```python
from build123d import *

# Parameters (mm, degrees)
SKETCH_1_R                  = 0.95
EXTRUDE_1_DEPTH             = 1.8
FILLET_1_R                  = 2
HOLE_WIZARD_M2_1_AT_2_COUNT = 2
HOLE_WIZARD_M2_1_AT_2_PITCH = 24
HOLE_WIZARD_M2_1_AT_3_COUNT = 2
HOLE_WIZARD_M2_1_AT_3_PITCH = 39.40177661
HOLE_WIZARD_M2_1_AT_4_COUNT = 2
HOLE_WIZARD_M2_1_AT_4_PITCH = 45
HOLE_WIZARD_M2_1_AT_5_COUNT = 2
HOLE_WIZARD_M2_1_AT_5_PITCH = 38.065732621
HOLE_WIZARD_M2_1_AT_6_COUNT = 2
HOLE_WIZARD_M2_1_AT_6_PITCH = 21.737065119
SKETCH_4_R                  = 17.25
SKETCH_4_R_2                = 15
EXTRUDE_2_DEPTH             = 4.2
SKETCH_4_2_R                = 15
CUT_EXTRUDE_2_DEPTH         = 3.5
SKETCH_7_R                  = 0.85
EXTRUDE_3_DEPTH             = 6
SKETCH_7_2_R                = 0.85
CUT_EXTRUDE_4_DEPTH         = 7
SKETCH_8_R                  = 4
CUT_EXTRUDE_5_DEPTH         = 10


with BuildPart() as part:
    # Sketch 1 → Extrude 1 (new body)
    with BuildSketch(Plane(origin=(0, 0, 0), x_dir=(1, 0, 0), z_dir=(0, 1, 0))):
        Polygon((33, 0), (16.5, 28.578838325), (-16.5, 28.578838325), (-33, 0), (-16.5, -28.578838325), (16.5, -28.578838325), align=None)
        with Locations(Location((-12, 19.032866311, 0), (0, 0, 270))):  # turned: the seam where the file's is
            Circle(SKETCH_1_R, mode=Mode.SUBTRACT)
        with Locations(Location((-12, -19.032866311, 0), (0, 0, 90))):  # turned: the seam where the file's is
            Circle(SKETCH_1_R, mode=Mode.SUBTRACT)
        with Locations(Location((-22.5, 0, 0), (0, 0, 270))):  # turned: the seam where the file's is
            Circle(SKETCH_1_R, mode=Mode.SUBTRACT)
        with Locations(Location((22.5, 0, 0), (0, 0, 90))):  # turned: the seam where the file's is
            Circle(SKETCH_1_R, mode=Mode.SUBTRACT)
        with Locations(Location((12, -19.032866311, 0), (0, 0, 270))):  # turned: the seam where the file's is
            Circle(SKETCH_1_R, mode=Mode.SUBTRACT)
        with Locations(Location((12, 19.032866311, 0), (0, 0, 90))):  # turned: the seam where the file's is
            Circle(SKETCH_1_R, mode=Mode.SUBTRACT)
    extrude(amount=EXTRUDE_1_DEPTH)

    # Fillet 1
    fillet_1_edges = [part.edges().sort_by_distance(p)[0] for p in [
        (16.5, 0.9, 28.578838325),
        (-16.5, 0.9, 28.578838325),
        (-33, 0.9, 0),
        (-16.5, 0.9, -28.578838325),
        (16.5, 0.9, -28.578838325),
        (33, 0.9, 0),
    ]]
    fillet(fillet_1_edges, radius=FILLET_1_R)

    # Sketch 3 → Hole Wizard M2 _1 (revolve, cut)
    with BuildSketch(Plane(origin=(12, 0, -19.032866311), x_dir=(0, 0, -1), z_dir=(1, 0, 0))):
        Polygon((0, 0), (0, 1.8), (0.9, 1.8), (0.9, 1.2), (2.1, 0), align=None)
    hole_wizard_m2_1 = revolve(axis=Axis((12, -6.35, -19.032866311), (0, 1, 0)), mode=Mode.SUBTRACT)

    # Hole Wizard M2 _1 at 2: Hole Wizard M2 _1 ×2
    with Locations(*[(-i * HOLE_WIZARD_M2_1_AT_2_PITCH, 0, 0) for i in range(1, HOLE_WIZARD_M2_1_AT_2_COUNT)]):
        add(hole_wizard_m2_1, mode=Mode.SUBTRACT)

    # Hole Wizard M2 _1 at 3: Hole Wizard M2 _1 ×2
    with Locations(*[Vector(-0.875595036, 0, 0.483045892) * (i * HOLE_WIZARD_M2_1_AT_3_PITCH) for i in range(1, HOLE_WIZARD_M2_1_AT_3_COUNT)]):
        add(hole_wizard_m2_1, mode=Mode.SUBTRACT)

    # Hole Wizard M2 _1 at 4: Hole Wizard M2 _1 ×2
    with Locations(*[Vector(-0.533333333, 0, 0.845905169) * (i * HOLE_WIZARD_M2_1_AT_4_PITCH) for i in range(1, HOLE_WIZARD_M2_1_AT_4_COUNT)]):
        add(hole_wizard_m2_1, mode=Mode.SUBTRACT)

    # Hole Wizard M2 _1 at 5: Hole Wizard M2 _1 ×2
    with Locations(*[(0, 0, i * HOLE_WIZARD_M2_1_AT_5_PITCH) for i in range(1, HOLE_WIZARD_M2_1_AT_5_COUNT)]):
        add(hole_wizard_m2_1, mode=Mode.SUBTRACT)

    # Hole Wizard M2 _1 at 6: Hole Wizard M2 _1 ×2
    with Locations(*[Vector(0.483045892, 0, 0.875595036) * (i * HOLE_WIZARD_M2_1_AT_6_PITCH) for i in range(1, HOLE_WIZARD_M2_1_AT_6_COUNT)]):
        add(hole_wizard_m2_1, mode=Mode.SUBTRACT)

    # Sketch 4 → Extrude 2 (add)
    with BuildSketch(Plane.XZ):
        with Locations(Location((0, 0, 0), (0, 0, 90))):  # turned: the seam where the file's is
            Circle(SKETCH_4_R)
        with Locations(Location((0, 0, 0), (0, 0, 270))):  # turned: the seam where the file's is
            Circle(SKETCH_4_R_2, mode=Mode.SUBTRACT)
    extrude(amount=EXTRUDE_2_DEPTH)

    # Sketch 4_2 → Cut-Extrude 2 (cut)
    with BuildSketch(Plane.XZ):
        with Locations(Location((0, 0, 0), (0, 0, 90))):  # turned: the seam where the file's is
            Circle(SKETCH_4_2_R)
    extrude(amount=-CUT_EXTRUDE_2_DEPTH, mode=Mode.SUBTRACT)

    # Sketch 7 → Extrude 3 (add)
    with BuildSketch(Plane.XZ.offset(4.2)):
        with BuildLine():
            ThreePointArc((-13.77195188, 10.387292305), (-9.652159983, 8.099123882), (-12.620960341, 11.758990606))
            ThreePointArc((-12.620960341, 11.758990606), (-13.214266644, 11.088086267), (-13.77195188, 10.387292305))
        make_face()
        with Locations((-11.490666647, 9.641814145)):
            Circle(SKETCH_7_R, mode=Mode.SUBTRACT)
        with BuildLine():
            ThreePointArc((13.77195188, 10.387292305), (9.652159983, 8.099123882), (12.620960341, 11.758990606))
            ThreePointArc((12.620960341, 11.758990606), (13.214266644, 11.088086267), (13.77195188, 10.387292305))
        make_face()
        with Locations((11.490666647, 9.641814145)):
            Circle(SKETCH_7_R, mode=Mode.SUBTRACT)
        with BuildLine():
            ThreePointArc((13.77195188, -10.387292305), (9.652159983, -8.099123882), (12.620960341, -11.758990606))
            ThreePointArc((12.620960341, -11.758990606), (13.214266644, -11.088086267), (13.77195188, -10.387292305))
        make_face()
        with Locations((11.490666647, -9.641814145)):
            Circle(SKETCH_7_R, mode=Mode.SUBTRACT)
        with BuildLine():
            ThreePointArc((-13.77195188, -10.387292305), (-9.652159983, -8.099123882), (-12.620960341, -11.758990606))
            ThreePointArc((-12.620960341, -11.758990606), (-13.214266644, -11.088086267), (-13.77195188, -10.387292305))
        make_face()
        with Locations((-11.490666647, -9.641814145)):
            Circle(SKETCH_7_R, mode=Mode.SUBTRACT)
    extrude(amount=-EXTRUDE_3_DEPTH)

    # Sketch 7_2 → Cut-Extrude 4 (cut, through all)
    with BuildSketch(Plane.XZ.offset(4.2)):
        with Locations(Location((-11.490666647, 9.641814145, 0), (0, 0, 270))):  # turned: the seam where the file's is
            Circle(SKETCH_7_2_R)
        with Locations(Location((11.490666647, 9.641814145, 0), (0, 0, 90))):  # turned: the seam where the file's is
            Circle(SKETCH_7_2_R)
        with Locations(Location((11.490666647, -9.641814145, 0), (0, 0, 270))):  # turned: the seam where the file's is
            Circle(SKETCH_7_2_R)
        with Locations(Location((-11.490666647, -9.641814145, 0), (0, 0, 90))):  # turned: the seam where the file's is
            Circle(SKETCH_7_2_R)
    extrude(amount=-CUT_EXTRUDE_4_DEPTH, mode=Mode.SUBTRACT)

    # Sketch 8 → Cut-Extrude 5 (cut)
    with BuildSketch(Plane(origin=(0, 1.8, 0), x_dir=(1, 0, 0), z_dir=(0, 1, 0))):
        with Locations(Location((-23.2, 0, 0), (0, 0, 270))):  # turned: the seam where the file's is
            Circle(SKETCH_8_R)
    extrude(amount=-CUT_EXTRUDE_5_DEPTH, mode=Mode.SUBTRACT)


solid = part.part
```
Work out the finished part from the listing and answer in its coordinate system (mm). A direction names the side the tool comes from. Coordinates: 2 decimals unless noted, no trailing zeros. Loops run counter-clockwise (first coordinate to the right, second up) from the corner with the lowest first, then second, coordinate; pieces in that order, holes last.
1) Flat-ended cylindrical pins translate along their axes: pin 1 (2.5 mm diameter, centred on x = 12, z = -19.03, fed in from -Y); pin 2 (2 mm diameter, centred on x = 22.5, z = 0, fed in from -Y); pin 3 (1.4 mm diameter, centred on x = -11.49, z = -9.64, fed in from -Y); pin 4 (3 mm diameter, centred on x = 7.5, y = -2, fed in from +Z). Find the tip coordinate at first contact, or state that the pin passes through.
Results:
pin 1: stops at y = 0.85
pin 2: stops at y = 1.1
pin 3: passes through
pin 4: stops at z = 16.17
2) For faces 5 (the cylindrical face through (16.36, 0.91, -28.3)), 6 (the flat face through (14, 0, 12)), 7 (the cylindrical face through (0, -1, -15)), determine the directions among +Z, -Z, +X, -X, +Y, -Y from which every point of the face is accessible in a straight line to the end or side of a thin tool.
Results:
face 5: -Z, +X, +Y, -Y
face 6: -Y
face 7: +Y, -Y
3) Section A-A (z = 13) is taken. Give the vertices of the cut face in (x, y), plus the area to 3 significant figures.
Results:
outline: (-25.49, 0) - (-11.34, 0) - (-11.34, -4.2) - (-7.48, -4.2) - (-7.48, 1.8) - (-25.49, 1.8) - close; (7.48, -4.2) - (11.34, -4.2) - (11.34, 0) - (25.49, 0) - (25.49, 1.8) - (7.48, 1.8) - close
area: 97.2 mm2
4) Section D-D (y = -2) is taken. Give the vertices of the cut face in (x, z), plus the area to 3 significant figures.
Results:
outline: circle Ø34.5 at (0, 0); hole (-12.88, -7.69) arc R2.4 cw to (-9.81, -11.35) arc R15 ccw to (9.81, -11.35) arc R2.4 cw to (12.88, -7.69) arc R15 ccw to (12.88, 7.69) arc R2.4 cw to (9.81, 11.35) arc R15 ccw to (-9.81, 11.35) arc R2.4 cw to (-12.88, 7.69) arc R15 ccw to start; hole circle Ø1.7 at (-11.49, -9.64); hole circle Ø1.7 at (-11.49, 9.64); hole circle Ø1.7 at (11.49, -9.64); hole circle Ø1.7 at (11.49, 9.64)
area: 254 mm2
5) Consider probe 1 along Z at (x, y) = (-0.5, -2.75); probe 2 along Z at (x, y) = (-12, 1.75); probe 3 along Y at (x, z) = (-14, -20.5). Determine where each line is inside the solid, lowest interval first.
Results:
probe 1: z = -17.24 to -14.99, 14.99 to 17.24
probe 2: z = -28.58 to -19.98, -18.08 to -10.32, -8.96 to -7.3, 7.3 to 8.96, 10.32 to 18.08, 19.98 to 28.58
probe 3: y = 0 to 1.8
6) Section C-C (z = 0) is taken. Give the vertices of the cut face in (x, y), plus the area to 3 significant figures.
Results:
outline: (-32.69, 0) - (-27.2, 0) - (-27.2, 1.8) - (-32.69, 1.8) - close; (-19.2, 0) - (-17.25, 0) - (-17.25, -4.2) - (-15, -4.2) - (-15, 1.8) - (-19.2, 1.8) - close; (15, -4.2) - (17.25, -4.2) - (17.25, 0) - (20.4, 0) - (21.55, 1.15) - (21.55, 1.8) - (15, 1.8) - close; (23.45, 1.15) - (24.6, 0) - (32.69, 0) - (32.69, 1.8) - (23.45, 1.8) - close
area: 63.4 mm2
7) Section B-B (x = -23.2) is taken. Give the vertices of the cut face in (y, z), plus the area to 3 significant figures.
Results:
outline: (0, -16.97) - (1.8, -16.97) - (1.8, -4) - (0, -4) - close; (0, 4) - (1.8, 4) - (1.8, 16.97) - (0, 16.97) - close
area: 46.7 mm2
8) For a pull along X with two mould halves and no side action, classify faces 1 (the cylindrical face through (-9.685, -1.242, -8.061)), 2 (the flat face through (10, -4.2, -9)), 3 (the cylindrical face through (16.36, 0.91, 28.3)), 4 (the cylindrical face through (-32.69, 0.91, -0.01)) as +X half, -X half, draft (parallel to the pull), parting line (faces both ways), or undercut.
Results:
face 1: undercut
face 2: draft
face 3: +X half
face 4: -X half
